from build123d import *

# Parameters (mm, degrees)
BOSS_EXTRUDE1_START = 31.75
SKETCH3_R           = 1.5875
BOSS_EXTRUDE1_DEPTH = 63.5
FILLET1_R           = 7.055555556
SKETCH5_W           = 16.383
SKETCH5_H           = 7.055555556
CUT_EXTRUDE1_DEPTH  = 43.200038063
LPATTERN1_COUNT     = 5
LPATTERN1_PITCH     = 14.111111111
FILLET2_R           = 1.175925926


with BuildPart() as part:
    # Sketch3 → Boss-Extrude1 (new body)
    with BuildSketch(Plane(origin=(0, 0, 0), x_dir=(1, 0, 0), z_dir=(0, 1, 0)).offset(BOSS_EXTRUDE1_START)):
        with BuildLine():
            Line((26.9875, 6.6675), (26.9875, 1.5875))
            Line((26.9875, 1.5875), (6.6675, 1.5875))
            Line((6.6675, 1.5875), (6.6675, 0))
            ThreePointArc((6.6675, 0), (-4.714634464, -4.714634464), (0, 6.6675))
            Line((0, 6.6675), (26.9875, 6.6675))
        make_face()
        with Locations(Location((0, 0, 0), (0, 0, 270))):
            Circle(SKETCH3_R, mode=Mode.SUBTRACT)
    extrude(amount=-BOSS_EXTRUDE1_DEPTH)

    # Fillet1
    fillet1_edges = [part.edges().sort_by_distance(p)[0] for p in [
        (26.9875, -31.75, -4.1275),
        (26.9875, 31.75, -4.1275),
    ]]
    fillet(fillet1_edges, radius=FILLET1_R)

    # Sketch5 → Cut-Extrude1 (cut, symmetric)
    with BuildSketch(Plane.XY):
        with Locations((0, 28.222222222)):
            Rectangle(SKETCH5_W, SKETCH5_H)
    cut_extrude1 = extrude(amount=CUT_EXTRUDE1_DEPTH, both=True, mode=Mode.SUBTRACT)

    # LPattern1: Cut-Extrude1 ×5
    with Locations(*[(0, -i * LPATTERN1_PITCH, 0) for i in range(1, LPATTERN1_COUNT)]):
        add(cut_extrude1, mode=Mode.SUBTRACT)

    # Fillet2
    fillet2_edges = [part.edges().sort_by_distance(p)[0] for p in [
        (8.1915, -3.527777778, -4.1275),
        (8.1915, 3.527777778, -4.1275),
        (8.1915, -17.638888889, -4.1275),
        (8.1915, -10.583333333, -4.1275),
        (8.1915, -24.694444444, -4.1275),
        (8.1915, 24.694444444, -4.1275),
        (8.1915, 10.583333333, -4.1275),
        (8.1915, 17.638888889, -4.1275),
    ]]
    fillet(fillet2_edges, radius=FILLET2_R)


solid = part.part
Verification items for the finished model (mm, model axes). A direction names the side the tool comes from. Round coordinates to 2 decimals unless told otherwise and drop trailing zeros. Loops run counter-clockwise (first coordinate to the right, second up) from the corner with the lowest first, then second, coordinate; pieces in that order, holes last. Notation, with made-up numbers: (6.5, 14) - (50.5, 14) arc R20 ccw to (50.5, 49) - close; hole circle Ø7 at (1.5, -18). An arc over 180 degrees is marked (long way). Answer in a Markdown table with one row per item. Add a question column.
Q1. Section check A-A on y = -18.5. Enter the section's corners in (x, z) (1 decimal).
Q2. Release check for a two-part mould opening along Y. For faces 5 (the face through (-0.966, 21.216, -1.26)), 6 (the face through (14, -31.75, -4)), 7 (the face through (2, -3.528, 0)), 8 (the face through (2, 24.694, 0)) record: pulls with the +Y half, pulls with the -Y half, needs draft (parallel to the pull), parting line crosses it, or undercut.
Q3. Section check D-D on y = 13. Enter the section's corners in (x, z).
Q4. Gauge pin test, flat ends, axial feed: pin 1 (4 mm diameter, centred on x = 0, z = 0, fed in from -Y); pin 2 (10 mm diameter, centred on x = 14.5, y = 2, fed in from +Z); pin 3 (5 mm diameter, centred on y = 14.5, z = -3.5, fed in from -X). Record the tip position at first contact, or that the pin passes through.
Q5. Tool access check on faces 1 (the face through (8.192, -29, -4)), 2 (the face through (6.668, 7, -1)), 3 (the face through (8.192, 29, -4)), 4 (the face through (7.84, -3.19, -4.09)). Record the directions out of +Z, -Z, +X, -X, +Y, -Y that give a thin tool (end or side, any length) a straight path to the whole face; none if there is none.
Q6. Section check C-C on x = 6. Enter the section's corners in (y, z), plus the area to 3 significant figures.
Q7. Section check B-B on z = 5.75. Enter the section's corners in (x, y), plus the area to 3 significant figures.
Q8. Material ranges on line 1 (Y direction, x = -4.5, z = -0.5); line 2 (X direction, y = -5.5, z = 0); line 3 (Z direction, x = 17.5, y = 16), recorded low to high.
Found:
| question | item | result |
|---|---|---|
| 1 | outline | (0, -6.7) - (27, -6.7) - (27, -1.6) - (6.7, -1.6) - (6.7, 0) arc R6.7 ccw (long way) to start; hole circle Ø3.2 at (0, 0) |
| 2 | face 5 | needs draft |
| 2 | face 6 | pulls with the -Y half |
| 2 | face 7 | undercut |
| 2 | face 8 | pulls with the +Y half |
| 3 | outline | (8.19, -6.67) - (26.99, -6.67) - (26.99, -1.59) - (8.19, -1.59) - close |
| 4 | pin 1 | stops at y = -24.69 |
| 4 | pin 2 | stops at z = -1.59 |
| 4 | pin 3 | stops at x = 8.06 |
| 5 | face 1 | +Z, -Z, -X, -Y |
| 5 | face 2 | +Z, +X, +Y, -Y |
| 5 | face 3 | +Z, -Z, -X, +Y |
| 5 | face 4 | +Z, -Z, -X |
| 6 | outline | (-24.69, -6.67) - (-17.64, -6.67) - (-17.64, 2.91) - (-24.69, 2.91) - close; (-10.58, -6.67) - (-3.53, -6.67) - (-3.53, 2.91) - (-10.58, 2.91) - close; (3.53, -6.67) - (10.58, -6.67) - (10.58, 2.91) - (3.53, 2.91) - close; (17.64, -6.67) - (24.69, -6.67) - (24.69, 2.91) - (17.64, 2.91) - close |
| 6 | area | 270 mm² |
| 7 | outline | (-3.38, -24.69) - (3.38, -24.69) - (3.38, -17.64) - (-3.38, -17.64) - close; (-3.38, -10.58) - (3.38, -10.58) - (3.38, -3.53) - (-3.38, -3.53) - close; (-3.38, 3.53) - (3.38, 3.53) - (3.38, 10.58) - (-3.38, 10.58) - close; (-3.38, 17.64) - (3.38, 17.64) - (3.38, 24.69) - (-3.38, 24.69) - close |
| 7 | area | 191 mm² |
| 8 | line 1 | y = -24.69 to -17.64, -10.58 to -3.53, 3.53 to 10.58, 17.64 to 24.69 |
| 8 | line 2 | x = -6.67 to -1.59, 1.59 to 6.67 |
| 8 | line 3 | z = -6.67 to -1.59 |
